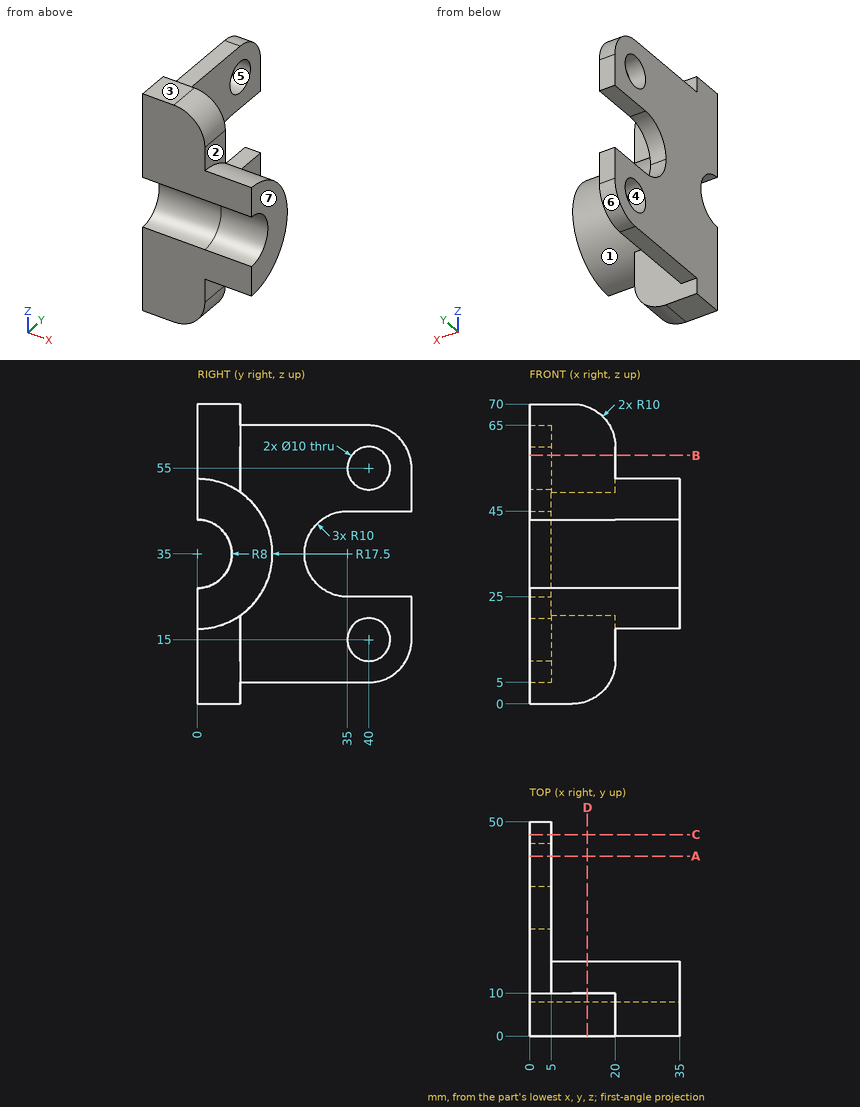
Design review of the part shown in the three views and the two pictorial views. Dimensions are in mm from the part's minimum x, y and z. A direction names the side the tool comes from. Round coordinates to 2 decimals unless told otherwise and drop trailing zeros. Loops run counter-clockwise (first coordinate to the right, second up) from the corner with the lowest first, then second, coordinate; pieces in that order, holes last. Notation, with made-up numbers: (-16.75, 73.25) -> (7.25, 73.25) arc R23 ccw to (7.25, 90.25) -> close; hole circle Ø10 at (12.5, -10.5). An arc over 180 degrees is marked (long way). Use one line per item in the form item = value. Start each with the question number.
Q1. Wall thickness on line 1 along Y through (x, z) = (3.1, 15); line 2 along X through (y, z) = (8.5, 59); line 3 along X through (y, z) = (31.5, 10): over which ranges is each line inside the solid? List them lowest first. Write a range as [from, to].
Q2. We need section C-C on y = 47. Give the boundary of the cut face in (x, z).
Q3. Machinability: for the marked faces 1, 2 and 3, which of the approach directions +Z, -Z, +X, -X, +Y, -Y give a long, thin tool a straight path to every point of the face, cutting with its end or side? Answer none if there is none.
Q4. For pin 1 Ø13 at (y, z) = (40, 15) entering from +X; pin 2 Ø1.5 at (x, y) = (30, 13) entering from +Z; pin 3 Ø6 at (x, z) = (11.5, 11.5) entering from +Y, all flat-tipped, find the tip position at first contact; note any pin that passes through.
Q5. We need section B-B on z = 58. Give the boundary of the cut face in (x, y), then the cut area to 3 significant figures.
Q6. Draft analysis for pull direction Z (two halves, no side actions). For the marked faces 4, 5, 6 and 7, state which applies: +Z half, -Z half, draft (parallel to the pull), parting line (faces both ways), or undercut.
Q7. We need section D-D on x = 13.5. Give the boundary of the cut face in (y, z).
Q8. We need section A-A on y = 42. Give the boundary of the cut face in (x, z).
Calculated:
q1.line_1 = [0, 35], [45, 50]
q1.line_2 = [0, 20]
q1.line_3 = [0, 5]
q2.outline = (0, 7.86) -> (5, 7.86) -> (5, 25) -> (0, 25) -> close; (0, 45) -> (5, 45) -> (5, 62.14) -> (0, 62.14) -> close
q3.face_1 = +X, +Y
q3.face_2 = +Z, +X, +Y
q3.face_3 = +Z, +X, -X, +Y, -Y
q4.pin_1 = 5
q4.pin_2 = 47.5
q4.pin_3 = 10
q5.outline = (0, 0) -> (20, 0) -> (20, 10) -> (5, 10) -> (5, 36) -> (0, 36) -> close; (0, 44) -> (5, 44) -> (5, 49.54) -> (0, 49.54) -> close
q5.area = 358 mm²
q6.face_4 = undercut
q6.face_5 = undercut
q6.face_6 = -Z half
q6.face_7 = draft
q7.outline = (0, 0.63) -> (10, 0.63) -> (10, 20.64) arc R17.5 ccw to (10, 49.36) -> (10, 69.37) -> (0, 69.37) -> (0, 43) arc R8 cw to (0, 27) -> close
q8.outline = (0, 5.2) -> (5, 5.2) -> (5, 10.42) -> (0, 10.42) -> close; (0, 19.58) -> (5, 19.58) -> (5, 25) -> (0, 25) -> close; (0, 45) -> (5, 45) -> (5, 50.42) -> (0, 50.42) -> close; (0, 59.58) -> (5, 59.58) -> (5, 64.8) -> (0, 64.8) -> close
